Can you work these out from the model? Positions are in its coordinate system, mm. Round coordinates to 2 decimals unless told otherwise and drop trailing zeros. Loops run counter-clockwise (first coordinate to the right, second up) from the corner with the lowest first, then second, coordinate; pieces in that order, holes last. Notation, with made-up numbers: M 55,-5 L 102,-5 A28 ccw 102,15 Z; hole C -3.5,2 d4. An arc over 180 degrees is marked long. Answer as CSV lines item,"result".
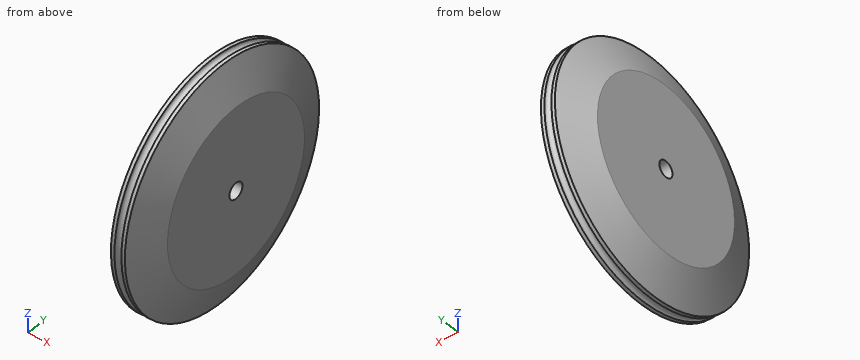
from build123d import *

# Parameters (mm, degrees)
F2_R     = 0.25
F4_R     = 0.575
F5_DEPTH = 3


with BuildPart() as f1:
    # F0 (on Front) → F1 (revolve)
    with BuildSketch(Plane.XZ):
        Polygon((-1.5, 0), (1.5, 0), (1.5, 6), (0.5, 8.5), (-0.5, 8.5), (-1.5, 6), align=None)
    revolve(axis=Axis((0, 0, 0), (-1, 0, 0)))

    # F2 (on Front) → F3 (revolve, cut)
    with BuildSketch(Plane.XZ):
        with Locations((0, 8.5)):
            Circle(F2_R)
    revolve(axis=Axis((0.73948, 0, 0), (1, 0, 0)), mode=Mode.SUBTRACT)

    # F4 (on face) → F5 (cut, through all)
    with BuildSketch(Plane.YZ.offset(1.5)):
        Circle(F4_R)
    extrude(amount=-F5_DEPTH, mode=Mode.SUBTRACT)


solid = f1.part
Item 1: Will this pin go through, and if not, where does the flat tip stop? pin 1 (1.5 mm diameter, centred on x = 0.5, y = 2, fed in from +Z).
Output:
pin 1,"stops at z = 8.41"
Item 2: If I drill on line 1 along Z through (x, y) = (0.3, 0) (3 decimals); line 2 along Z through (x, y) = (0.3, -0.5); line 3 along Y through (x, z) = (0.1, -1.25), over which ranges is the centre line in solid material (lowest first)? Write a range as from..to.
Output:
line 1,"z = -8.5..-0.575, 0.575..8.5"
line 2,"z = -8.49..-0.28, 0.28..8.49"
line 3,"y = -8.18..8.18"
Item 3: If we section it at D-D on x = 1.1: Write out the boundary of the cut face in (y, z) (3 decimals).
Output:
outline,"C 0,0 d14; hole C 0,0 d1.15"
Item 4: If we section it at A-A on z = 0: Write out the boundary of the cut face in (x, y) (3 decimals), then the cut area to 3 significant figures.
Output:
outline,"M -1.5,-6 L -0.5,-8.5 L -0.25,-8.5 A0.25 cw 0.25,-8.5 L 0.5,-8.5 L 1.5,-6 L 1.5,-0.575 L -1.5,-0.575 Z; M -1.5,0.575 L 1.5,0.575 L 1.5,6 L 0.5,8.5 L 0.25,8.5 A0.25 cw -0.25,8.5 L -0.5,8.5 L -1.5,6 Z"
area,"42.4 mm2"
Item 5: If we section it at C-C on x = -0.8: Write out the boundary of the cut face in (y, z) (3 decimals).
Output:
outline,"C 0,0 d15.5; hole C 0,0 d1.15"
